Input: dimensioned drawing with shaded views. Units: mm. Origin: part minimum x, y, z. Round coordinates to 2 decimals unless told otherwise and drop trailing zeros. Loops run counter-clockwise (first coordinate to the right, second up) from the corner with the lowest first, then second, coordinate; pieces in that order, holes last. Notation, with made-up numbers: M -32.75,58.5 L -8.75,58.5 A19 cw -8.75,65.5 Z; hole C -10.5,86.5 d8. An arc over 180 degrees is marked long. Write each question's results on one line, items separated by ' | '. Start each with the question number.
1. Section A-A on x = 511. Output: boundary loops of the cut face in (y, z), and give its area (3 significant figures).
2. Ray query, line 1 (Y direction, x = 759, z = 38.5) (1 decimal); line 2 (Y direction, x = 445.5, z = 731); line 3 (X direction, y = 195.5, z = 312.5) (1 decimal). Return the intervals inside material, ascending.
3. Contact query for flat-ended pins moving along their axis: pin 1 Ø1 at (x, y) = (860, 232) entering from +Z (1 decimal); pin 2 Ø3 at (y, z) = (391, 588) entering from -X (1 decimal); pin 3 Ø10 at (x, z) = (839, 100.5) entering from -Y. Output: stop coordinate, or through.
4. Section B-B on y = 436. Output: boundary loops of the cut face in (x, z) (1 decimal).
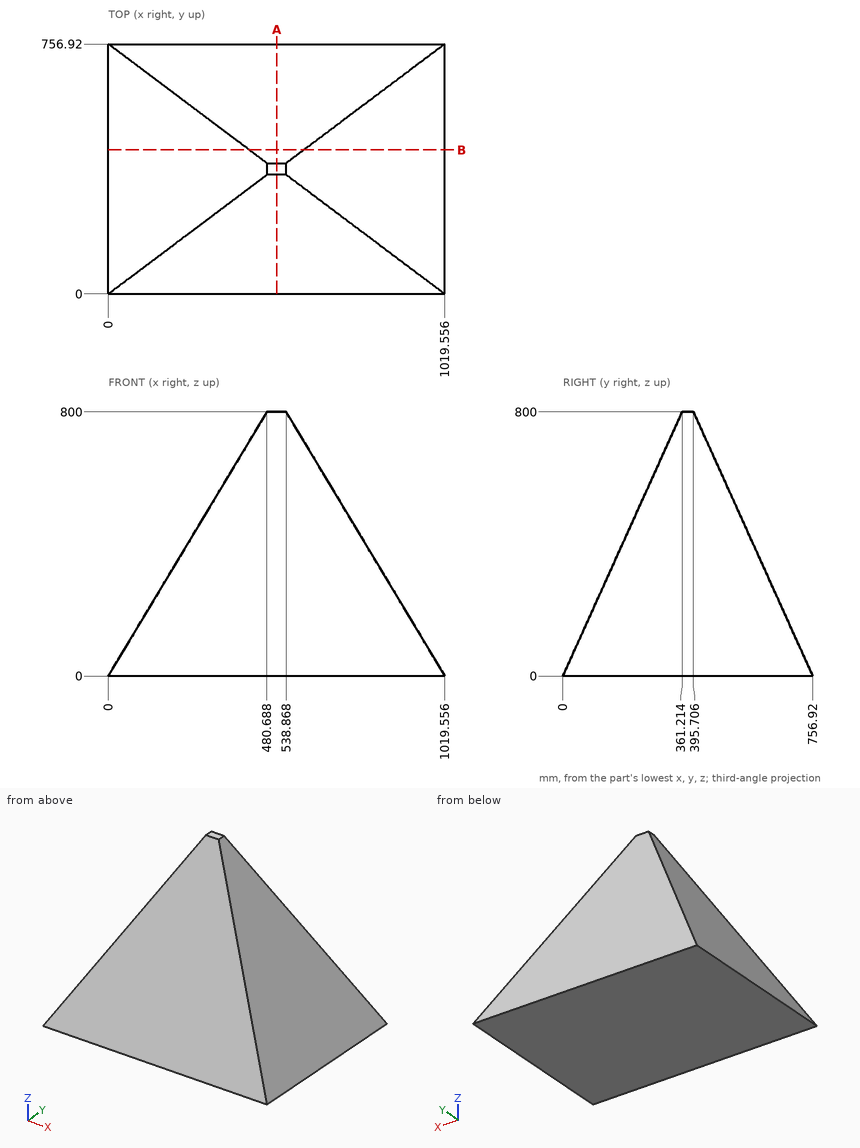
Taken from the geometry:
1) outline: M 0,0 L 756.92,0 L 395.71,800 L 361.21,800 Z | area: 317,000 mm^2
2) line 1: 17.4 to 739.5 | line 2: 330.06 to 426.86 | line 3: 187.8 to 831.8
3) pin 1: z = 266.4 | pin 2: x = 352.4 | pin 3: y = 43.12
4) outline: M 0,0 L 1019.6,0 L 592.5,710.8 L 427.1,710.8 Z
